from build123d import *

# Parameters (mm, degrees)
SZKIC1_R                    = 28
DODANIE_WYCI_GNI_CIE1_DEPTH = 6
SZKIC3_R                    = 22.5
WYTNIJ_WYCI_GNI_CIE1_DEPTH  = 6
SZKIC5_R                    = 4.5
DODANIE_WYCI_GNI_CIE2_DEPTH = 6
SZKIC6_R                    = 1.55
WYTNIJ_WYCI_GNI_CIE2_DEPTH  = 6


with BuildPart() as part:
    # Szkic1 → Dodanie-wyciągnięcie1 (new body)
    with BuildSketch(Plane.XY):
        with Locations((51.52186297, 19.852107637)):
            Circle(SZKIC1_R)
    extrude(amount=DODANIE_WYCI_GNI_CIE1_DEPTH)

    # Szkic3 → Wytnij-wyciągnięcie1 (cut)
    with BuildSketch(Plane.XY.offset(6)):
        with Locations((51.52186297, 19.852107637)):
            Circle(SZKIC3_R)
    extrude(amount=-WYTNIJ_WYCI_GNI_CIE1_DEPTH, mode=Mode.SUBTRACT)

    # Szkic5 → Dodanie-wyciągnięcie2 (add)
    with BuildSketch(Plane.XY.offset(6)):
        with Locations((78.52186297, 19.852107638)):
            Circle(SZKIC5_R)
        with Locations((38.02186297, -3.530578265)):
            Circle(SZKIC5_R)
        with Locations((38.02186297, 43.23479354)):
            Circle(SZKIC5_R)
    extrude(amount=-DODANIE_WYCI_GNI_CIE2_DEPTH)

    # Szkic6 → Wytnij-wyciągnięcie2 (cut)
    with BuildSketch(Plane.XY.offset(6)):
        with Locations((78.52186297, 19.852107638)):
            Circle(SZKIC6_R)
        with Locations((38.02186297, -3.530578265)):
            Circle(SZKIC6_R)
        with Locations((38.02186297, 43.23479354)):
            Circle(SZKIC6_R)
    extrude(amount=-WYTNIJ_WYCI_GNI_CIE2_DEPTH, mode=Mode.SUBTRACT)


solid = part.part
Source: CAD feature listing. Evaluate the final solid. Frame: model axes, mm. Give positions to 0.01 mm unless a question says otherwise; leave off trailing zeros. Write each loop counter-clockwise with the first axis right and the second up, starting at its lowest first coordinate (ties: lowest second). Pieces come first, ordered by that corner, then holes. Notation, with made-up numbers: M 48,20 L 71,20 A20 cw 71,34 Z; hole C 26,-11 d4. An arc over 180 degrees is marked long. Answer as a JSON object with one key per item and string values.
Q1. Cut plane C-C, the plane y = 11.5. Return the cut outline in (x, z).
Geometry check:
{"outline": "M 24.8,0 L 30.63,0 L 30.63,6 L 24.8,6 Z; M 72.41,0 L 78.25,0 L 78.25,6 L 72.41,6 Z"}
Q2. Cut plane A-A, the plane y = 19. Return the cut outline in (x, z), then the cut area to 3 significant figures.
Geometry check:
{"outline": "M 23.53,0 L 29.04,0 L 29.04,6 L 23.53,6 Z; M 74.01,0 L 77.23,0 L 77.23,6 L 74.01,6 Z; M 79.82,0 L 82.94,0 L 82.94,6 L 79.82,6 Z", "area": "71.1 mm^2"}
Q3. Ray query, line 1 along X through (y, z) = (18.5, 4.9); line 2 along X through (y, z) = (33, 1); line 3 along X through (y, z) = (14.5, 5). Return the intervals inside material, ascending.
Geometry check:
{"line 1": "x = 23.55 to 29.06, 73.98 to 77.76, 79.28 to 82.81", "line 2": "x = 26.8 to 33.26, 69.78 to 76.24", "line 3": "x = 24.04 to 29.67, 73.38 to 79.01"}
Q4. Cut plane D-D, the plane z = 0.95. Return the cut outline in (x, y), then the cut area to 3 significant figures.
Geometry check:
{"outline": "M 33.84,-1.86 A4.5 ccw 41.56,-6.31 A28 ccw 79.17,15.4 A4.5 ccw 79.17,24.31 A28 ccw 41.56,46.02 A4.5 ccw 33.84,41.57 A28 ccw Z; hole C 51.52,19.85 d45; hole C 38.02,-3.53 d3.1; hole C 38.02,43.23 d3.1; hole C 78.52,19.85 d3.1", "area": "922 mm^2"}
Q5. Mould query, pull axis Y, two halves, no side actions, for faces 1 (the face through (63.618, 38.824, 3.042)), 2 (the face through (65.22, -4.57, 2.96)), 3 (the face through (36, 3, 0)), 4 (the face through (83.02, 19.76, 3.04)). Classes: +Y half, -Y half, draft (parallel to the pull), parting line (faces both ways), or undercut.
Geometry check:
{"face 1": "undercut", "face 2": "-Y half", "face 3": "draft", "face 4": "parting line"}
Q6. Contact query for flat-ended pins moving along their axis: P1, Ø1.9, axis at x = 38.02, y = 43.23, coming from the +Z side; P2, Ø3, axis at y = 12.5, z = 5, coming from the +X side; P3, Ø1.5, axis at x = 46, z = 3.5, coming from the +Y side; P4, Ø1, axis at y = -0.5, z = 1, coming from the +X side. Output: stop coordinate, or through.
Geometry check:
{"P1": "passes through", "P2": "stops at x = 78.9", "P3": "stops at y = 47.44", "P4": "stops at x = 71.27"}
Q7. Cut plane B-B, the plane x = 61. Return the cut outline in (y, z).
Geometry check:
{"outline": "M -6.49,0 L -0.55,0 L -0.55,6 L -6.49,6 Z; M 40.26,0 L 46.2,0 L 46.2,6 L 40.26,6 Z"}
